Can you work these out from the model? Positions are in its coordinate system, mm. Face numbers are marked on the shaded views. A direction names the side the tool comes from. Round coordinates to 2 decimals unless told otherwise and drop trailing zeros. Order: outer loops, then holes, each group sorted by start corner. A loop starts at its lowest first (then second) coordinate and runs counter-clockwise, first axis right, second up. Notation, with made-up numbers: (35, 15) -> (49, 15) arc R24 cw to (49, 26) -> close; hole circle Ø4 at (-2, 28.25). An arc over 180 degrees is marked (long way). One line per item, written item: value.
```python
from build123d import *

# Parameters (mm, degrees)
SKETCH1_W           = 80
SKETCH1_H           = 80
BOSS_EXTRUDE1_DEPTH = 20
CUT_EXTRUDE1_DEPTH  = 21
SKETCH3_R           = 24
CUT_EXTRUDE2_DEPTH  = 21
CUT_EXTRUDE3_DEPTH  = 21
SKETCH5_R           = 6
CUT_EXTRUDE4_DEPTH  = 81
FILLET1_R           = 4


with BuildPart() as part:
    # Sketch1 → Boss-Extrude1 (new body)
    with BuildSketch(Plane.XY):
        with Locations((40, 40)):
            Rectangle(SKETCH1_W, SKETCH1_H)
    extrude(amount=-BOSS_EXTRUDE1_DEPTH)

    # Sketch2 → Cut-Extrude1 (cut, through all)
    with BuildSketch(Plane.XY):
        Polygon((16, 0), (64, 0), (64, 12), (70, 12), (70, 36), (10, 36), (10, 12), (16, 12), align=None)
    extrude(amount=-CUT_EXTRUDE1_DEPTH, mode=Mode.SUBTRACT)

    # Sketch3 → Cut-Extrude2 (cut, through all)
    with BuildSketch(Plane.XY):
        with Locations((40, 36)):
            Circle(SKETCH3_R)
    extrude(amount=-CUT_EXTRUDE2_DEPTH, mode=Mode.SUBTRACT)

    # Sketch4 → Cut-Extrude3 (cut, through all)
    with BuildSketch(Plane.XY):
        with BuildLine():
            Line((4, 36), (0, 36))
            Line((0, 36), (0, 80))
            Line((0, 80), (28, 80))
            Line((28, 80), (28, 69.941125497))
            ThreePointArc((28, 69.941125497), (10.606123087, 56.784609691), (4, 36))
        make_face()
        with BuildLine():
            Line((76, 36), (80, 36))
            Line((80, 36), (80, 80))
            Line((80, 80), (52, 80))
            Line((52, 80), (52, 69.941125497))
            ThreePointArc((52, 69.941125497), (69.393876913, 56.784609691), (76, 36))
        make_face()
    extrude(amount=-CUT_EXTRUDE3_DEPTH, mode=Mode.SUBTRACT)

    # Sketch5 → Cut-Extrude4 (cut, through all)
    with BuildSketch(Plane(origin=(0, 80, 0), x_dir=(1, 0, 0), z_dir=(0, 1, 0))):
        with Locations((40, 10)):
            Circle(SKETCH5_R)
    extrude(amount=-CUT_EXTRUDE4_DEPTH, mode=Mode.SUBTRACT)

    # Fillet1
    fillet1_edges = [part.edges().sort_by_distance(p)[0] for p in [
        (76, 36, -10),
        (52, 69.941125497, -10),
        (28, 69.941125497, -10),
        (4, 36, -10),
    ]]
    fillet(fillet1_edges, radius=FILLET1_R)


solid = part.part
```
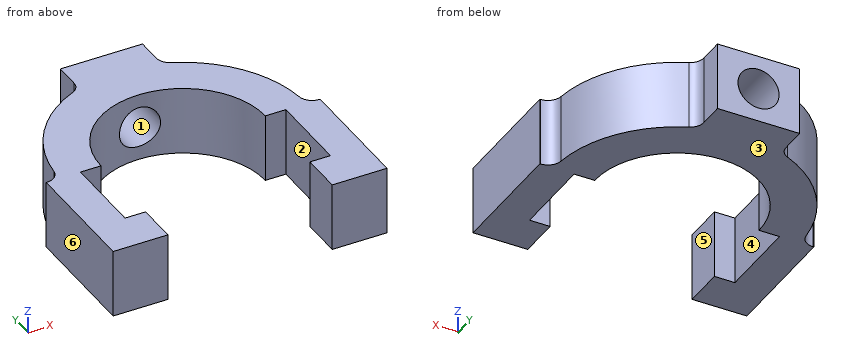
Q1. Please list where these lines run through material, in increasing order: line 1 along X through (y, z) = (22, -5); line 2 along Z through (x, y) = (40, 74); line 3 along X through (y, z) = (75, -10).
Answers below:
line 1: 0 to 10, 70 to 80
line 2: -20 to -16, -4 to 0
line 3: 28 to 34, 46 to 52
Q2. Will these pins go through, and if not, where does the flat tip stop? pin 1 Ø5 at (y, z) = (19.5, -4.5) entering from -X; pin 2 Ø5 at (x, z) = (66, -7) entering from +Y; pin 3 Ø1.5 at (y, z) = (65, -10.5) entering from +X; pin 4 Ø6 at (y, z) = (76.5, -6) entering from +X.
Answers below:
pin 1: x = 0
pin 2: y = 63.27
pin 3: x = 62.31
pin 4: x = 52
Q3. We'd pull the mould along Z, two halves only. Please class the marked faces 1, 2 and 3: released by +Z, released by -Z, zero draft, split by the parting line, or undercut.
Answers below:
face 1: undercut
face 2: zero draft
face 3: released by -Z
Q4. I want a section at C-C on z = -10. List the corners of the cut face in (x, y) for me, plus the area to 3 significant figures.
Answers below:
outline: (0, 0) -> (16, 0) -> (16, 12) -> (10, 12) -> (10, 36) -> (16, 36) arc R24 cw to (34, 59.24) -> (34, 80) -> (28, 80) -> (28, 72.66) arc R4 cw to (25.6, 68.99) arc R36 ccw to (4.18, 39.6) arc R4 cw to (0.2, 36) -> (0, 36) -> close; (46, 59.24) arc R24 cw to (64, 36) -> (70, 36) -> (70, 12) -> (64, 12) -> (64, 0) -> (80, 0) -> (80, 36) -> (79.8, 36) arc R4 cw to (75.82, 39.6) arc R36 ccw to (54.4, 68.99) arc R4 cw to (52, 72.66) -> (52, 80) -> (46, 80) -> close
area: 1,970 mm^2
Q5. I want a section at A-A on y = 25. List the corners of the cut face in (x, z) for me, plus the area to 3 significant figures.
Answers below:
outline: (0, -20) -> (10, -20) -> (10, 0) -> (0, 0) -> close; (70, -20) -> (80, -20) -> (80, 0) -> (70, 0) -> close
area: 400 mm^2
Q6. On a 3-axis mill with a long thin cutter (end or side, diameter ignored), from which of +Z, -Z, +X, -X, +Y, -Y can I reach the whole of each face in a straight line? I mean the marked faces 4, 5 and 6. Say none if no direction works.
Answers below:
face 4: +Z, -Z
face 5: +Z, -Z, -Y
face 6: +Z, -Z, -X, +Y, -Y
Q7. I want a section at D-D on y = 74.5. List the corners of the cut face in (x, z) for me, plus the area to 3 significant figures.
Answers below:
outline: (28, -20) -> (52, -20) -> (52, 0) -> (28, 0) -> close; hole circle Ø12 at (40, -10)
area: 367 mm^2
Q8. I want a section at B-B on x = 40. List the corners of the cut face in (y, z) for me.
Answers below:
outline: (60, -20) -> (80, -20) -> (80, -16) -> (60, -16) -> close; (60, -4) -> (80, -4) -> (80, 0) -> (60, 0) -> close
